from build123d import *

# Parameters (mm, degrees)
CROQUIS22_W                        = 100
CROQUIS22_H                        = 90
BRIDA_BASE4_DEPTH                  = 3.175
BRIDA_DE_ARISTA1_STRIP_W           = 14.1732
BRIDA_DE_ARISTA1_STRIP_H           = 3.175
BRIDA_DE_ARISTA1_STRIP_CUT_DEPTH   = 90
BRIDA_DE_ARISTA1_STRIP_2_W         = 14.1732
BRIDA_DE_ARISTA1_STRIP_2_H         = 3.175
BRIDA_DE_ARISTA1_STRIP_CUT_2_DEPTH = 90
BRIDA_DE_ARISTA1_DEPTH             = 90
BRIDA_DE_ARISTA1_BEND_DEPTH        = 90
CROQUIS33_R                        = 8
CROQUIS33_R_2                      = 3.5
CORTAR_EXTRUIR3_DEPTH              = 14.7625
CROQUIS35_R                        = 13
CROQUIS35_R_2                      = 2.5
CORTAR_EXTRUIR4_DEPTH              = 14.7625
CROQUIS36_R                        = 17.5
CORTAR_EXTRUIR5_DEPTH              = 14.7625
CROQUIS37_R                        = 4.5
CROQUIS37_R_2                      = 30
CORTAR_EXTRUIR6_DEPTH              = 14.7625
REDONDEO1_R                        = 40
CROQUIS40_R                        = 2.5
CORTAR_EXTRUIR7_DEPTH              = 14.7625


# Sheet-metal steps are written as plain solids
with BuildPart() as part:
    # Croquis22 → Brida base4 (new body)
    with BuildSketch(Plane.XY):
        Rectangle(CROQUIS22_W, CROQUIS22_H)
    extrude(amount=-BRIDA_BASE4_DEPTH)

    # Brida de arista1 strip (across the edge) → Brida de arista1 strip cut (cut)
    with BuildSketch(Plane(origin=(-50, 45, 0), x_dir=(1, 0, 0), z_dir=(0, -1, 0))):
        with Locations((-3.175, -1.5875)):
            Rectangle(BRIDA_DE_ARISTA1_STRIP_W, BRIDA_DE_ARISTA1_STRIP_H)
    extrude(amount=BRIDA_DE_ARISTA1_STRIP_CUT_DEPTH, mode=Mode.SUBTRACT)

    # Brida de arista1 strip 2 (across the edge) → Brida de arista1 strip cut 2 (cut)
    with BuildSketch(Plane(origin=(50, -45, 0), x_dir=(-1, 0, 0), z_dir=(0, 1, 0))):
        with Locations((-3.175, -1.5875)):
            Rectangle(BRIDA_DE_ARISTA1_STRIP_2_W, BRIDA_DE_ARISTA1_STRIP_2_H)
    extrude(amount=BRIDA_DE_ARISTA1_STRIP_CUT_2_DEPTH, mode=Mode.SUBTRACT)

    # Brida de arista1 section (across the edge) → Brida de arista1 (add)
    with BuildSketch(Plane(origin=(-50, 45, 0), x_dir=(1, 0, 0), z_dir=(0, -1, 0))):
        with BuildLine():
            Line((0, 0.7366), (0, 66.825))
            Line((0, 66.825), (3.175, 66.825))
            Line((3.175, 66.825), (3.175, 0.7366))
            ThreePointArc((3.175, 0.7366), (3.390745145, 0.215745145), (3.9116, 0))
            Line((3.9116, 0), (3.9116, -3.175))
            ThreePointArc((3.9116, -3.175), (1.145681115, -2.029318885), (0, 0.7366))
        make_face()
    extrude(amount=BRIDA_DE_ARISTA1_DEPTH)

    # Brida de arista1 section 2 (across the edge) → Brida de arista1 bend (add)
    with BuildSketch(Plane(origin=(50, -45, 0), x_dir=(-1, 0, 0), z_dir=(0, 1, 0))):
        with BuildLine():
            Line((0, 0.7366), (0, 66.825))
            Line((0, 66.825), (3.175, 66.825))
            Line((3.175, 66.825), (3.175, 0.7366))
            ThreePointArc((3.175, 0.7366), (3.390745145, 0.215745145), (3.9116, 0))
            Line((3.9116, 0), (3.9116, -3.175))
            ThreePointArc((3.9116, -3.175), (1.145681115, -2.029318885), (0, 0.7366))
        make_face()
    extrude(amount=BRIDA_DE_ARISTA1_BEND_DEPTH)

    # Croquis33 → Cortar-Extruir3 (cut)
    with BuildSketch(Plane.ZY.offset(50)):
        with Locations((33.7808, 0)):
            Circle(CROQUIS33_R)
        with Locations((12.7808, 18.5)):
            Circle(CROQUIS33_R_2)
        with Locations((12.7808, -18.5)):
            Circle(CROQUIS33_R_2)
    extrude(amount=-CORTAR_EXTRUIR3_DEPTH, mode=Mode.SUBTRACT)

    # Croquis35 → Cortar-Extruir4 (cut)
    with BuildSketch(Plane(origin=(50, 0, 0), x_dir=(0, 0, -1), z_dir=(1, 0, 0))):
        with Locations((-33.7808, 0)):
            Circle(CROQUIS35_R)
        with Locations((-33.7808, 17.5)):
            Circle(CROQUIS35_R_2)
        with Locations((-33.7808, -17.5)):
            Circle(CROQUIS35_R_2)
        with Locations((-16.2808, 0)):
            Circle(CROQUIS35_R_2)
        with Locations((-51.2808, 0)):
            Circle(CROQUIS35_R_2)
    extrude(amount=-CORTAR_EXTRUIR4_DEPTH, mode=Mode.SUBTRACT)

    # Croquis36 → Cortar-Extruir5 (cut)
    with BuildSketch(Plane.ZY.offset(50)):
        with Locations((33.7808, 0)):
            Circle(CROQUIS36_R)
    extrude(amount=-CORTAR_EXTRUIR5_DEPTH, mode=Mode.SUBTRACT)

    # Croquis37 → Cortar-Extruir6 (cut)
    with BuildSketch(Plane.XY):
        with Locations((-30, 28.181524588)):
            Circle(CROQUIS37_R)
        with Locations((-30, -28.621860909)):
            Circle(CROQUIS37_R)
        with Locations((30, 28.181524588)):
            Circle(CROQUIS37_R)
        with Locations((30, -28.621860909)):
            Circle(CROQUIS37_R)
        Circle(CROQUIS37_R_2)
    extrude(amount=-CORTAR_EXTRUIR6_DEPTH, mode=Mode.SUBTRACT)

    # Redondeo1
    redondeo1_edges = [part.edges().sort_by_distance(p)[0] for p in [
        (-48.4125, 45, 66.825),
        (-48.4125, -45, 66.825),
        (48.4125, -45, 66.825),
        (48.4125, 45, 66.825),
    ]]
    fillet(redondeo1_edges, radius=REDONDEO1_R)

    # Croquis40 → Cortar-Extruir7 (cut)
    with BuildSketch(Plane(origin=(50, 0, 0), x_dir=(0, 0, -1), z_dir=(1, 0, 0))):
        with Locations((-5.7366, 35)):
            Circle(CROQUIS40_R)
        with Locations((-5.7366, -35)):
            Circle(CROQUIS40_R)
    extrude(amount=-CORTAR_EXTRUIR7_DEPTH, mode=Mode.SUBTRACT)


solid = part.part
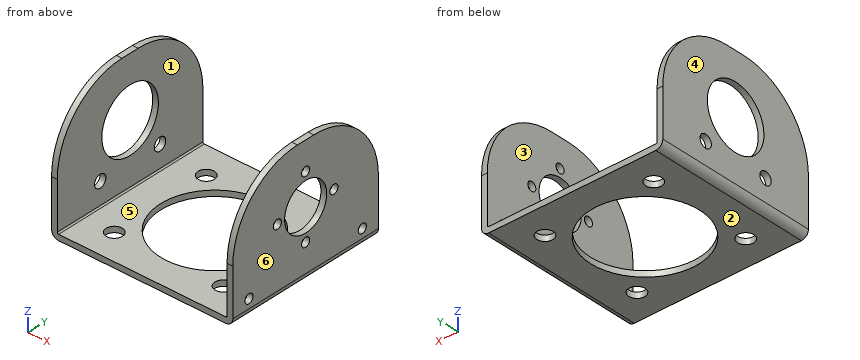
Read the model definition and answer for the solid it produces. Units are mm, in the model's axes. Face numbers are marked on the shaded views. A direction names the side the tool comes from. Coordinates: 2 decimals unless noted, no trailing zeros. Loops run counter-clockwise (first coordinate to the right, second up) from the corner with the lowest first, then second, coordinate; pieces in that order, holes last.
Q1. Which of the six approach directions +Z, -Z, +X, -X, +Y, -Y give full straight-line access (tool end or side, diameter ignored) to the marked faces 1 and 2?
Q2. The part is cut by section C-C on z = 15. Write down the section's boundary in (x, y) (1 decimal), and give its area (3 significant figures).
Q3. The mould has two halves that part along X. Classify the marked faces 3, 4, 5 and 6: +X half, -X half, draft (parallel to the pull), parting line (faces both ways), or undercut.
Q4. The part is cut by section B-B on y = 0. Give the number of separate pieces and of enclosed holes in the cut face, and give its area (3 significant figures).
Q5. Each of these flat-tipped pins is pushed along its axis until it touches: pin 1 Ø3 at (x, y) = (-5, 28.5) entering from +Z; pin 2 Ø23.5 at (y, z) = (0, 33.78) entering from +X (3 decimals); pin 3 Ø6.5 at (y, z) = (-18.5, 12.78) entering from -X (3 decimals); pin 4 Ø3 at (y, z) = (35, 5.74) entering from +X (3 decimals). Where does it stop, or does it pass through?
Q6. The part is cut by section A-A on x = 0. Write down the section's boundary in (y, z) (3 decimals).
Q7. Consider probe 1 along X at (y, z) = (-28, 42) (3 decimals); probe 2 along X at (y, z) = (-2, 51.5) (3 decimals); probe 3 along Z at (x, y) = (-46, -12.5) (3 decimals). Determine where each line is inside the solid, lowest interval first.
Q8. The part is cut by section D-D on z = 40.5. Write down the section's boundary in (x, y) (3 decimals), and give its area (3 significant figures).
Results below:
1. face 1: +Z, +Y, -Y
1. face 2: -Z, +X, -X, +Y, -Y
2. outline: (-50, -45) - (-46.8, -45) - (-46.8, -21.2) - (-50, -21.2) - close; (-50, -15.8) - (-46.8, -15.8) - (-46.8, 15.8) - (-50, 15.8) - close; (-50, 21.2) - (-46.8, 21.2) - (-46.8, 45) - (-50, 45) - close; (46.8, -45) - (50, -45) - (50, -2.1) - (46.8, -2.1) - close; (46.8, 2.1) - (50, 2.1) - (50, 45) - (46.8, 45) - close
2. area: 523 mm2
3. face 3: undercut
3. face 4: -X half
3. face 5: undercut
3. face 6: +X half
4. separate pieces: 6
4. enclosed holes: 0
4. area: 320 mm2
5. pin 1: stops at z = 0
5. pin 2: passes through
5. pin 3: stops at x = 46.825
5. pin 4: stops at x = -46.825
6. outline: (-45, -3.175) - (-30, -3.175) - (-30, 0) - (-45, 0) - close; (30, -3.175) - (45, -3.175) - (45, 0) - (30, 0) - close
7. probe 1: x = -50 to -46.825, 46.825 to 50
7. probe 2: x = -50 to -46.825
7. probe 3: z = -3.175 to 0
8. outline: (-50, -42.59) - (-46.825, -42.59) - (-46.825, -16.159) - (-50, -16.159) - close; (-50, 16.159) - (-46.825, 16.159) - (-46.825, 42.59) - (-50, 42.59) - close; (46.825, -42.59) - (50, -42.59) - (50, -11.129) - (46.825, -11.129) - close; (46.825, 11.129) - (50, 11.129) - (50, 42.59) - (46.825, 42.59) - close
8. area: 368 mm2
